Here's how the part is built. I have some questions about the finished solid (model axes, mm). A direction names the side the tool comes from. Give positions to 0.01 mm unless a question says otherwise; leave off trailing zeros. Loops run counter-clockwise (first coordinate to the right, second up) from the corner with the lowest first, then second, coordinate; pieces in that order, holes last. Notation, with made-up numbers: (42.25, -23.5) - (64.25, -23.5) arc R16 ccw to (64.25, -6.5) - close; hole circle Ø1 at (69, 64.25). An arc over 180 degrees is marked (long way). Use a Markdown table: item, result.
from build123d import *

# Parameters (mm, degrees)
BOSS_EXTRUDE1_DEPTH     = 200
CUT_EXTRUDE1_DEPTH      = 208.419799276
CUT_EXTRUDE1_DEPTH_BACK = 208.419799276
BODY_CUT_W              = 190
BODY_CUT_H              = 45
SCREW_HOLES_R           = 3.05778
SCREW_HOLES_R_2         = 1.7645
CUT_EXTRUDE9_DEPTH      = 10


with BuildPart() as part:
    # body sketch → Boss-Extrude1 (new body)
    with BuildSketch(Plane.XY):
        with BuildLine():
            Line((-11.792788403, 31.296564203), (-7.835417036, 31.296564203))
            ThreePointArc((-7.835417036, 31.296564203), (-7.367491329, 31.168035209), (-6.937848459, 30.94246665))
            Line((-6.937848459, 30.94246665), (-3.083381198, 27.087999388))
            Line((-3.083381198, 27.087999388), (-3.083381198, 26.62720762))
            ThreePointArc((-3.083381198, 26.62720762), (-3.247157606, 26.33019226), (-3.544172966, 26.166415852))
            Line((-3.544172966, 26.166415852), (-6.093887415, 26.166415852))
            ThreePointArc((-6.093887415, 26.166415852), (-6.684013327, 25.91258072), (-6.937848459, 25.322454808))
            Line((-6.937848459, 25.322454808), (-6.937848459, 23.771246138))
            ThreePointArc((-6.937848459, 23.771246138), (-6.853833412, 23.540250894), (-6.645828951, 23.409287254))
            Line((-6.645828951, 23.409287254), (22.5, 23.409287254))
            Line((22.5, 23.409287254), (22.5, -31.590712746))
            Line((22.5, -31.590712746), (-22.5, -31.590712746))
            Line((-22.5, -31.590712746), (-22.5, 23.409287254))
            Line((-22.5, 23.409287254), (-12.982376489, 23.409287254))
            ThreePointArc((-12.982376489, 23.409287254), (-12.774372027, 23.540250894), (-12.69035698, 23.771246138))
            Line((-12.69035698, 23.771246138), (-12.69035698, 25.322454808))
            ThreePointArc((-12.69035698, 25.322454808), (-12.944192112, 25.91258072), (-13.534318024, 26.166415852))
            Line((-13.534318024, 26.166415852), (-16.084032474, 26.166415852))
            ThreePointArc((-16.084032474, 26.166415852), (-16.381047834, 26.33019226), (-16.544824242, 26.62720762))
            Line((-16.544824242, 26.62720762), (-16.544824242, 27.087999388))
            Line((-16.544824242, 27.087999388), (-12.69035698, 30.94246665))
            ThreePointArc((-12.69035698, 30.94246665), (-12.260714111, 31.168035209), (-11.792788403, 31.296564203))
        make_face()
    extrude(amount=BOSS_EXTRUDE1_DEPTH)

    # body cut → Cut-Extrude1 (cut, two sides: drawn at the far end of the back side and taken through both)
    with BuildSketch(Plane(origin=(22.5, 0, 0), x_dir=(0, 0, -1), z_dir=(1, 0, 0)).offset(-CUT_EXTRUDE1_DEPTH_BACK)):
        with Locations((-100, -4.090712746)):
            Rectangle(BODY_CUT_W, BODY_CUT_H)
    extrude(amount=CUT_EXTRUDE1_DEPTH + CUT_EXTRUDE1_DEPTH_BACK, mode=Mode.SUBTRACT)

    # screw holes → Cut-Extrude9 (cut)
    with BuildSketch(Plane(origin=(0, -31.590712746, 0), x_dir=(-1, 0, 0), z_dir=(0, -1, 0))):
        with Locations(Location((-0.7, -100, 0), (0, 0, 90))):
            Circle(SCREW_HOLES_R)
        with Locations(Location((-0.696336872, -81.999941546, 0), (0, 0, 90))):
            Circle(SCREW_HOLES_R_2)
        with Locations(Location((-0.696336872, -117.999941546, 0), (0, 0, 90))):
            Circle(SCREW_HOLES_R_2)
    extrude(amount=-CUT_EXTRUDE9_DEPTH, mode=Mode.SUBTRACT)


solid = part.part
(1) On a 3-axis mill with a long thin cutter (end or side, diameter ignored), from which of +Z, -Z, +X, -X, +Y, -Y can I reach the whole of each face in a straight line? I mean faces 5 (the face through (1.23, -29.13, 116.32)), 6 (the face through (0, 0, 0)), 7 (the face through (-18, 23.409, 99)), 8 (the face through (0, -4, 195)). Say none if no direction works.
A:
| item | result |
|---|---|
| face 5 | -Y |
| face 6 | -Z, +X, -X, +Y, -Y |
| face 7 | +Z, -Z, -X |
| face 8 | +X, -X |
(2) Will these pins go through, and if not, where does the flat tip stop? pin 1 (8 mm diameter, centred on x = 6, z = 169, fed in from +Y); pin 2 (0.5 mm diameter, centred on y = 25, z = 116.5, fed in from +X); pin 3 (0.8 mm diameter, centred on y = 25, z = 90, fed in from -X).
A:
| item | result |
|---|---|
| pin 1 | y = 23.41 |
| pin 2 | x = -6.94 |
| pin 3 | x = -12.7 |
(3) Suppose I cut it at C-C on y = 9.5. Write out the boundary of the cut face in (x, z), plus the area to 3 significant figures.
A:
| item | result |
|---|---|
| outline | (-22.5, 0) - (22.5, 0) - (22.5, 5) - (-22.5, 5) - close; (-22.5, 195) - (22.5, 195) - (22.5, 200) - (-22.5, 200) - close |
| area | 450 mm2 |
(4) If I drill on line 1 (Z direction, x = 9, y = -6); line 2 (Y direction, x = 14.5, z = 87); line 3 (Y direction, x = -10.5, z = 127), over which ranges is the centre line in solid material (lowest first)?
A:
| item | result |
|---|---|
| line 1 | 0 to 5, 195 to 200 |
| line 2 | -31.59 to -26.59, 18.41 to 23.41 |
| line 3 | -31.59 to -26.59, 18.41 to 31.3 |
(5) Suppose I cut it at B-B on x = 16.5. Write out the boundary of the cut face in (y, z), plus the area to 3 significant figures.
A:
| item | result |
|---|---|
| outline | (-31.59, 0) - (23.41, 0) - (23.41, 200) - (-31.59, 200) - close; hole (-26.59, 5) - (18.41, 5) - (18.41, 195) - (-26.59, 195) - close |
| area | 2,450 mm2 |
(6) Suppose I cut it at D-D on z = 136.5. Write out the boundary of the cut face in (x, y), plus the area to 3 significant figures.
A:
| item | result |
|---|---|
| outline | (-22.5, -31.59) - (22.5, -31.59) - (22.5, -26.59) - (-22.5, -26.59) - close; (-22.5, 18.41) - (22.5, 18.41) - (22.5, 23.41) - (-6.65, 23.41) arc R0.38 cw to (-6.94, 23.77) - (-6.94, 25.32) arc R0.87 cw to (-6.09, 26.17) - (-3.54, 26.17) arc R0.61 ccw to (-3.08, 26.63) - (-3.08, 27.09) - (-6.94, 30.94) arc R2.26 ccw to (-7.84, 31.3) - (-11.79, 31.3) arc R2.26 ccw to (-12.69, 30.94) - (-16.54, 27.09) - (-16.54, 26.63) arc R0.61 ccw to (-16.08, 26.17) - (-13.53, 26.17) arc R0.87 cw to (-12.69, 25.32) - (-12.69, 23.77) arc R0.38 cw to (-12.98, 23.41) - (-22.5, 23.41) - close |
| area | 517 mm2 |
(7) We'd pull the mould along X, two halves only. Please class faces 1 (the face through (-5, -26.591, 101)), 2 (the face through (1.89, -29.13, 83.3)), 3 (the face through (22.5, 20, 70)), 4 (the face through (-22.5, -27, 77)): pulls with the +X half, pulls with the -X half, needs draft (parallel to the pull), parting line crosses it, or undercut.
A:
| item | result |
|---|---|
| face 1 | needs draft |
| face 2 | undercut |
| face 3 | pulls with the +X half |
| face 4 | pulls with the -X half |
(8) Suppose I cut it at A-A on z = 100. Count the separate pieces of the cut face and the enclosed holes in it, plus the area to 3 significant figures.
A:
| item | result |
|---|---|
| separate pieces | 3 |
| enclosed holes | 0 |
| area | 487 mm2 |
